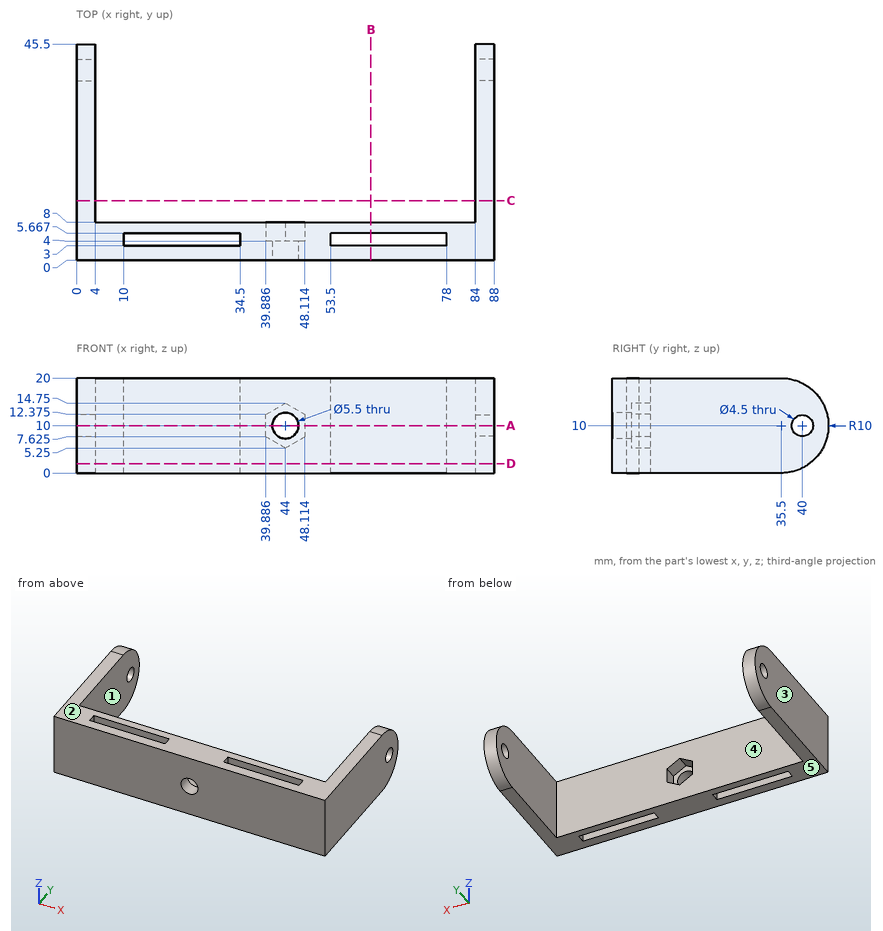
Design review of the part shown in the three views and the two pictorial views. Dimensions are in mm from the part's minimum x, y and z. A direction names the side the tool comes from. Give positions to 0.01 mm unless a question says otherwise; leave off trailing zeros. Loops run counter-clockwise (first coordinate to the right, second up) from the corner with the lowest first, then second, coordinate; pieces in that order, holes last. Notation, with made-up numbers: (4.5, 76) -> (40.5, 76) arc R22 cw to (40.5, 108) -> close; hole circle Ø8 at (-32, 11.25). An arc over 180 degrees is marked (long way). Put each result on its own line as item: value. Start each with the question number.
1. We need section B-B on x = 62. State the section outline as (y, z) points, then the cut area to 3 significant figures.
2. Mouldability with a two-part tool opening along X and no side actions: class the marked faces 3, 4 and 5 as released by +X, released by -X, zero draft, split by the parting line, or undercut.
3. For the marked faces 1 and 2, list the 3-axis set-ups (+Z, -Z, +X, -X, +Y, -Y) from which the entire face can be reached by the end or side of a thin tool; tool diameter is ignored.
4. We need section C-C on y = 12.5. State the section outline as (x, z) points, then the cut area to 3 significant figures.
5. Wall thickness on probe 1 along Y at (x, z) = (63.5, 19); probe 2 along X at (y, z) = (35.5, 9); probe 3 along Z at (x, y) = (44, 2): over which ranges is each line inside the solid? List them lowest first.
6. We need section D-D on z = 2. State the section outline as (x, y) points.
7. We need section A-A on z = 10. State how many separate pieces and enclosed holes the cut face has.
8. Clearance check with a flat-ended pin moving along its axis: P1, Ø10, axis at x = 71.5, z = 8, coming from the +Y side. State where the tip first meets the part, or that it passes through.
Determined:
1. outline: (0, 0) -> (3, 0) -> (3, 20) -> (0, 20) -> close; (5.67, 0) -> (8, 0) -> (8, 20) -> (5.67, 20) -> close
1. area: 107 mm^2
2. face 3: released by -X
2. face 4: undercut
2. face 5: zero draft
3. face 1: +Z, -Z, +Y
3. face 2: +Z, +X, -X, +Y, -Y
4. outline: (0, 0) -> (4, 0) -> (4, 20) -> (0, 20) -> close; (84, 0) -> (88, 0) -> (88, 20) -> (84, 20) -> close
4. area: 160 mm^2
5. probe 1: 0 to 3, 5.67 to 8
5. probe 2: 0 to 4, 84 to 88
5. probe 3: 0 to 7.25, 12.75 to 20
6. outline: (0, 0) -> (88, 0) -> (88, 41.5) -> (84, 41.5) -> (84, 8) -> (4, 8) -> (4, 41.5) -> (0, 41.5) -> close; hole (10, 3) -> (34.5, 3) -> (34.5, 5.67) -> (10, 5.67) -> close; hole (53.5, 3) -> (78, 3) -> (78, 5.67) -> (53.5, 5.67) -> close
7. separate pieces: 4
7. enclosed holes: 2
8. P1: y = 8
